```python
from build123d import *

# Parameters (mm, degrees)
SKETCH1_W           = 11
SKETCH1_H           = 11
BOSS_EXTRUDE1_DEPTH = 3.7
FILLET1_R           = 1
SKETCH2_W           = 3.85
SKETCH2_H           = 3.85
CUT_EXTRUDE1_DEPTH  = 2
SKETCH4_R           = 2.2
BOSS_EXTRUDE2_DEPTH = 2
BOSS_EXTRUDE3_DEPTH = 2
SKETCH3_R           = 1.2
CUT_EXTRUDE2_DEPTH  = 16.90565937
CUT_EXTRUDE3_DEPTH  = 16.303267625


with BuildPart() as part:
    # Sketch1 → Boss-Extrude1 (new body)
    with BuildSketch(Plane(origin=(0, 0, 0), x_dir=(1, 0, 0), z_dir=(0, 1, 0))):
        Rectangle(SKETCH1_W, SKETCH1_H)
    extrude(amount=BOSS_EXTRUDE1_DEPTH)

    # Fillet1
    fillet1_edges = [part.edges().sort_by_distance(p)[0] for p in [
        (5.5, 1.85, 5.5),
        (-5.5, 1.85, 5.5),
        (-5.5, 1.85, -5.5),
        (5.5, 1.85, -5.5),
    ]]
    fillet(fillet1_edges, radius=FILLET1_R)

    # Sketch2 → Cut-Extrude1 (cut)
    with BuildSketch(Plane(origin=(0, 3.7, 0), x_dir=(1, 0, 0), z_dir=(0, 1, 0))):
        with Locations((-2.825, 0)):
            Rectangle(SKETCH2_W, SKETCH2_H)
        with Locations((2.825, 0)):
            Rectangle(SKETCH2_W, SKETCH2_H)
    extrude(amount=-CUT_EXTRUDE1_DEPTH, mode=Mode.SUBTRACT)

    # Sketch4 → Boss-Extrude2 (add)
    with BuildSketch(Plane(origin=(0, 0, 0), x_dir=(-1, 0, 0), z_dir=(0, -1, 0))):
        with Locations(Location((2.825, 0, 0), (0, 0, 90))):
            Circle(SKETCH4_R)
        with Locations(Location((-2.825, 0, 0), (0, 0, 90))):
            Circle(SKETCH4_R)
    extrude(amount=BOSS_EXTRUDE2_DEPTH)

    # Sketch5 → Boss-Extrude3 (add)
    with BuildSketch(Plane(origin=(0, -2, 0), x_dir=(-1, 0, 0), z_dir=(0, -1, 0))):
        with BuildLine():
            Line((9.5, 10.5), (-9.5, 10.5))
            ThreePointArc((-9.5, 10.5), (-10.207106781, 10.207106781), (-10.5, 9.5))
            Line((-10.5, 9.5), (-10.5, -9.5))
            ThreePointArc((-10.5, -9.5), (-10.207106781, -10.207106781), (-9.5, -10.5))
            Line((-9.5, -10.5), (9.5, -10.5))
            ThreePointArc((9.5, -10.5), (10.207106781, -10.207106781), (10.5, -9.5))
            Line((10.5, -9.5), (10.5, 9.5))
            ThreePointArc((10.5, 9.5), (10.207106781, 10.207106781), (9.5, 10.5))
        make_face()
    extrude(amount=-BOSS_EXTRUDE3_DEPTH)

    # Sketch3 → Cut-Extrude2 (cut, through all)
    with BuildSketch(Plane(origin=(0, 3.7, 0), x_dir=(1, 0, 0), z_dir=(0, 1, 0))):
        with Locations(Location((-2.825, 0, 0), (0, 0, 270))):
            Circle(SKETCH3_R)
        with Locations(Location((2.825, 0, 0), (0, 0, 270))):
            Circle(SKETCH3_R)
    extrude(amount=-CUT_EXTRUDE2_DEPTH, mode=Mode.SUBTRACT)

    # Sketch7 → Cut-Extrude3 (cut, through all)
    with BuildSketch(Plane(origin=(0, 0, 0), x_dir=(1, 0, 0), z_dir=(0, 1, 0))):
        with BuildLine():
            Line((0, -9.085786438), (1.414213562, -10.5))
            Line((1.414213562, -10.5), (3.889087297, -8.025126266))
            ThreePointArc((3.889087297, -8.025126266), (4.035533906, -7.671572875), (3.889087297, -7.318019485))
            Line((3.889087297, -7.318019485), (3.181980515, -6.610912703))
            ThreePointArc((3.181980515, -6.610912703), (2.828427125, -6.464466094), (2.474873734, -6.610912703))
            Line((2.474873734, -6.610912703), (0, -9.085786438))
        make_face()
        with BuildLine():
            Line((-3.889087297, -8.025126266), (-1.414213562, -10.5))
            Line((-1.414213562, -10.5), (0, -9.085786438))
            Line((0, -9.085786438), (-2.474873734, -6.610912703))
            ThreePointArc((-2.474873734, -6.610912703), (-2.828427125, -6.464466094), (-3.181980515, -6.610912703))
            Line((-3.181980515, -6.610912703), (-3.889087297, -7.318019485))
            ThreePointArc((-3.889087297, -7.318019485), (-4.035533906, -7.671572875), (-3.889087297, -8.025126266))
        make_face()
        Polygon((-1.414213562, -10.5), (1.414213562, -10.5), (0, -9.085786438), align=None)
    extrude(amount=-CUT_EXTRUDE3_DEPTH, mode=Mode.SUBTRACT)


solid = part.part
```
Geometry: final body of the model. Coordinates: model frame, mm. A direction names the side the tool comes from. Round coordinates to 2 decimals unless told otherwise and drop trailing zeros. Order: outer loops, then holes, each group sorted by start corner. A loop starts at its lowest first (then second) coordinate and runs counter-clockwise, first axis right, second up. Notation, with made-up numbers: M -21,32 L 18,32 A22 ccw 18,59 Z; hole C -2.75,43 d7. An arc over 180 degrees is marked long. One line per item, written item: value.
(1) Pull-direction query (Z, two-part tool) for faces 4 (the flat face through (4.75, 3, 0)), 5 (the cylindrical face through (5.199, 1.876, 5.215)), 6 (the flat face through (0, -2, 0)); classes: pulls with the +Z half, pulls with the -Z half, needs draft (parallel to the pull), parting line crosses it, or undercut.
Result sheet:
face 4: undercut
face 5: pulls with the +Z half
face 6: needs draft
(2) Cut plane C-C (x = -8.75). Return the cut outline in (y, z).
Result sheet:
outline: M -2,-10.5 L 0,-10.5 L 0,10.5 L -2,10.5 Z
(3) Reachability of faces 1 (the flat face through (-1.22, -0.986, 7.866)), 2 (the cylindrical face through (-5.215, 1.876, -5.199)), 3 (the cylindrical face through (-5.215, 1.876, 5.199)) from +Z, -Z, +X, -X, +Y, -Y: full face, straight path, thin tool, end or side. Return the list, or none.
Result sheet:
face 1: +Y, -Y
face 2: -Z, -X, +Y
face 3: +Z, -X, +Y
(4) Pin query (flat end, axial travel): P1, Ø3, axis at x = 3.5, z = -0.5, coming from the +Y side; P2, Ø3, axis at x = 0.5, y = 2, coming from the -Z side; P3, Ø0.6, axis at y = 3, z = 0, coming from the -X side; P4, Ø1, axis at x = -2.5, y = 2, coming from the +Z side. Return the tip coordinate at first contact, or that it passes through.
Result sheet:
P1: y = 3.7
P2: z = -5.5
P3: x = -5.5
P4: z = 5.5
(5) Cut plane A-A (z = 0). Return the cut outline in (x, y) (3 decimals), and give its area (3 significant figures).
Result sheet:
outline: M -10.5,-2 L -4.025,-2 L -4.025,1.7 L -4.75,1.7 L -4.75,3.7 L -5.5,3.7 L -5.5,0 L -10.5,0 Z; M -1.625,-2 L 1.625,-2 L 1.625,1.7 L 0.9,1.7 L 0.9,3.7 L -0.9,3.7 L -0.9,1.7 L -1.625,1.7 Z; M 4.025,-2 L 10.5,-2 L 10.5,0 L 5.5,0 L 5.5,3.7 L 4.75,3.7 L 4.75,1.7 L 4.025,1.7 Z
area: 49.5 mm2
(6) Cut plane D-D (y = 0.35). Return the cut outline in (x, z) (3 decimals), and give its area (3 significant figures).
Result sheet:
outline: M -5.5,-4.5 A1 ccw -4.5,-5.5 L 4.5,-5.5 A1 ccw 5.5,-4.5 L 5.5,4.5 A1 ccw 4.5,5.5 L -4.5,5.5 A1 ccw -5.5,4.5 Z; hole C -2.825,0 d2.4; hole C 2.825,0 d2.4
area: 111 mm2
(7) Cut plane B-B (y = 3). Return the cut outline in (x, z) (3 decimals), and give its area (3 significant figures).
Result sheet:
outline: M -5.5,-4.5 A1 ccw -4.5,-5.5 L 4.5,-5.5 A1 ccw 5.5,-4.5 L 5.5,4.5 A1 ccw 4.5,5.5 L -4.5,5.5 A1 ccw -5.5,4.5 Z; hole M -4.75,-1.925 L -0.9,-1.925 L -0.9,1.925 L -4.75,1.925 Z; hole M 0.9,-1.925 L 4.75,-1.925 L 4.75,1.925 L 0.9,1.925 Z
area: 90.5 mm2
(8) Line query: probe 1 along X at (y, z) = (2.45, -1.5); probe 2 along X at (y, z) = (-0.5, 0) (3 decimals); probe 3 along Z at (x, y) = (4.25, 2.55) (3 decimals). Output: solid intervals per line, ascending. Write a range as [from, to].
Result sheet:
probe 1: [-5.5, -4.75], [-0.9, 0.9], [4.75, 5.5]
probe 2: [-10.5, -4.025], [-1.625, 1.625], [4.025, 10.5]
probe 3: [-5.5, -1.925], [1.925, 5.5]
